Could you check a few things on this model? Use its own coordinates, in mm. Face numbers are marked on the shaded views. A direction names the side the tool comes from. Give positions to 0.01 mm unless a question says otherwise; leave off trailing zeros. Order: outer loops, then holes, each group sorted by start corner. A loop starts at its lowest first (then second) coordinate and runs counter-clockwise, first axis right, second up. Notation, with made-up numbers: (52.25, 70) -> (73.25, 70) arc R20 cw to (73.25, 109) -> close; hole circle Ø5 at (86, -9.75). An arc over 180 degrees is marked (long way). Answer as CSV lines item,"result". Start each with the question number.
(1) I need wall thicknesses on L1, parallel to Z at x = -2.5, y = 6; L2, parallel to Y at x = -6.25, z = 15.25. Which ranges of each line are inside material? Lowest first, please.
(2) I want a section at B-B (z = 10.25). Please give me the cut outline in (x, y).
(3) I want a section at C-C (y = 8). Please give me the cut outline in (x, z), plus the area to 3 significant figures.
(4) I want a section at A-A (x = -2). Please give me the cut outline in (y, z), plus the area to 3 significant figures.
(5) Will this pin go through, and if not, where does the flat tip stop? pin 1 Ø4.5 at (x, y) = (-1.5, 13) entering from +Z.
(6) On a 3-axis mill with a long thin cutter (end or side, diameter ignored), from which of +Z, -Z, +X, -X, +Y, -Y can I reach the whole of each face in a straight line? I mean the marked faces 1 and 2. Say none if no direction works.
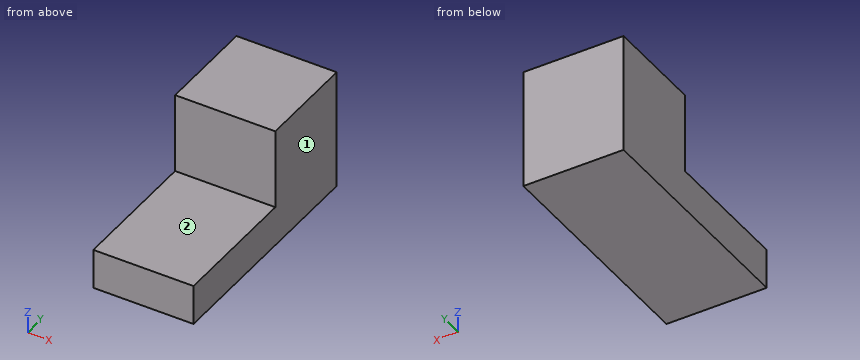
Solid Edge part; units mm, degrees
sketch "Sketch1" plane through (0, 0, 0) normal (1, 0, 0) x (0, 1, 0)
  line L0 (0, 0) -> (35, 0)
  line L1 (35, 0) -> (35, 18)
  line L2 (35, 18) -> (20, 18)
  line L3 (20, 18) -> (20, 6)
  line L4 (20, 6) -> (0, 6)
  line L5 (0, 6) -> (0, 0)
  dimension "D1" = 35
  dimension "D2" = 20
  dimension "D3" = 35
extrude "Protrusion1" add sketch "Sketch1" along normal mid plane 15
properties material "Polyethylene, low density"
Final values:
1,L1,"0 to 6"
1,L2,"20 to 35"
2,outline,"(-7.5, 20) -> (7.5, 20) -> (7.5, 35) -> (-7.5, 35) -> close"
3,outline,"(-7.5, 0) -> (7.5, 0) -> (7.5, 6) -> (-7.5, 6) -> close"
3,area,"90.0 mm²"
4,outline,"(0, 0) -> (35, 0) -> (35, 18) -> (20, 18) -> (20, 6) -> (0, 6) -> close"
4,area,"390 mm²"
5,pin 1,"z = 6"
6,face 1,"+Z, -Z, +X, +Y, -Y"
6,face 2,"+Z, +X, -X, -Y"
